Part model, mm, in its own coordinate system. Face numbers are marked on the shaded views. A direction names the side the tool comes from. Coordinates: 2 decimals unless noted, no trailing zeros. Order: outer loops, then holes, each group sorted by start corner. A loop starts at its lowest first (then second) coordinate and runs counter-clockwise, first axis right, second up.
1) Pin check, flat tips, straight feed: pin 1 Ø1.5 at (y, z) = (-3, 64) entering from +X; pin 2 Ø3 at (x, y) = (-2.5, -2.5) entering from +Z; pin 3 Ø1.5 at (y, z) = (9, 65) entering from -X. Stop position of each tip, or through.
2) Cut at B-B (z = 16). List the corners of the cut face in (x, y), and give its area (3 significant figures).
3) Mould opens along Z. For the marked faces 1, 2 and 3 say: +Z half, -Z half, draft (parallel to the pull), parting line (faces both ways), or undercut.
4) Cut at A-A (x = -23.5). List the corners of the cut face in (y, z), and give its area (3 significant figures).
5) Cut at C-C (y = 0). List the corners of the cut face in (x, z).
6) Tool access for the marked faces 4 and 5: list every direction of +Z, -Z, +X, -X, +Y, -Y with a clear straight run to the whole face (end or side of a thin tool).
7) Wall check: L1, parallel to Y at x = 18, z = -2.3; L2, parallel to X at y = 7.5, z = 4; L3, parallel to Z at x = 12, y = -9. Give the ranges that are in metal, low to high.
8) Cut at D-D (x = 18). List the corners of the cut face in (y, z).
```python
from build123d import *

# Parameters (mm, degrees)
SKETCH1_W                  = 50
SKETCH1_H                  = 50
BASE_FLANGE1_DEPTH         = 3
EDGE_FLANGE1_DEPTH         = 50
EDGE_FLANGE2_DEPTH         = 50
EDGE_FLANGE3_DEPTH         = 50
EDGE_FLANGE4_DEPTH         = 50
F_6_0_204_DIAMETER_SLOT1_D = 5.1816


# Sheet-metal steps are written as plain solids
with BuildPart() as part:
    # Sketch1 → Base-Flange1 (new body)
    with BuildSketch(Plane.XY):
        Rectangle(SKETCH1_W, SKETCH1_H)
    extrude(amount=-BASE_FLANGE1_DEPTH)

    # Edge-Flange1 section (across the edge) → Edge-Flange1 (add)
    with BuildSketch(Plane(origin=(28, -25, 0), x_dir=(-1, 0, 0), z_dir=(0, 1, 0))):
        with BuildLine():
            Line((-3, 3), (-3, 60))
            Line((-3, 60), (0, 60))
            Line((0, 60), (0, 3))
            ThreePointArc((0, 3), (0.878679656, 0.878679656), (3, 0))
            Line((3, 0), (3, -3))
            ThreePointArc((3, -3), (-1.242640687, -1.242640687), (-3, 3))
        make_face()
    extrude(amount=EDGE_FLANGE1_DEPTH)

    # Edge-Flange2 section (across the edge) → Edge-Flange2 (add)
    with BuildSketch(Plane(origin=(-28, 25, 0), x_dir=(1, 0, 0), z_dir=(0, -1, 0))):
        with BuildLine():
            Line((-3, 3), (-3, 60))
            Line((-3, 60), (0, 60))
            Line((0, 60), (0, 3))
            ThreePointArc((0, 3), (0.878679656, 0.878679656), (3, 0))
            Line((3, 0), (3, -3))
            ThreePointArc((3, -3), (-1.242640687, -1.242640687), (-3, 3))
        make_face()
    extrude(amount=EDGE_FLANGE2_DEPTH)

    # Edge-Flange3 section (across the edge) → Edge-Flange3 (add)
    with BuildSketch(Plane(origin=(-28, 25, 63), x_dir=(0, 0, -1), z_dir=(0, -1, 0))):
        with BuildLine():
            Line((-3, 3), (-3, 17))
            Line((-3, 17), (0, 17))
            Line((0, 17), (0, 3))
            ThreePointArc((0, 3), (0.878679656, 0.878679656), (3, 0))
            Line((3, 0), (3, -3))
            ThreePointArc((3, -3), (-1.242640687, -1.242640687), (-3, 3))
        make_face()
    extrude(amount=EDGE_FLANGE3_DEPTH)

    # Edge-Flange4 section (across the edge) → Edge-Flange4 (add)
    with BuildSketch(Plane(origin=(28, -25, 63), x_dir=(0, 0, -1), z_dir=(0, 1, 0))):
        with BuildLine():
            Line((-3, 3), (-3, 17))
            Line((-3, 17), (0, 17))
            Line((0, 17), (0, 3))
            ThreePointArc((0, 3), (0.878679656, 0.878679656), (3, 0))
            Line((3, 0), (3, -3))
            ThreePointArc((3, -3), (-1.242640687, -1.242640687), (-3, 3))
        make_face()
    extrude(amount=EDGE_FLANGE4_DEPTH)

    # #6 (0.204) Diameter Slot1 (through all)
    with Locations(Plane.XY.offset(66)):
        with Locations((-18, 15), (-18, -15), (18, 15), (18, -15)):
            Hole(F_6_0_204_DIAMETER_SLOT1_D / 2)


solid = part.part
```
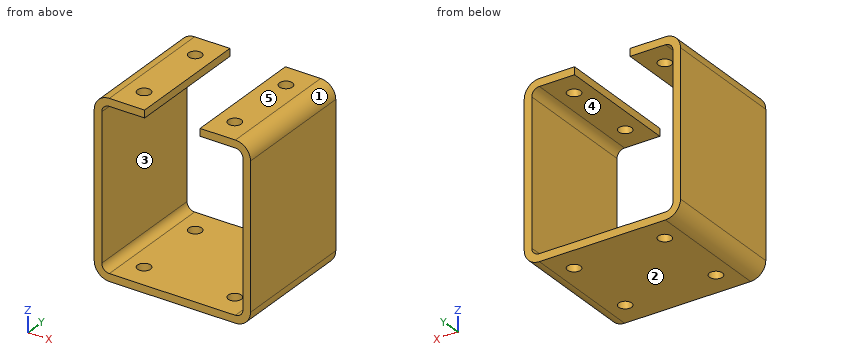
Geometry check:
1. pin 1: stops at x = 30.04
1. pin 2: stops at z = 0
1. pin 3: stops at x = -29.24
2. outline: (-31, -25) - (-28, -25) - (-28, 25) - (-31, 25) - close; (28, -25) - (31, -25) - (31, 25) - (28, 25) - close
2. area: 300 mm2
3. face 1: +Z half
3. face 2: -Z half
3. face 3: undercut
4. outline: (-25, -3) - (25, -3) - (25, 0) - (-25, 0) - close; (-25, 63) - (25, 63) - (25, 66) - (-25, 66) - close
4. area: 300 mm2
5. outline: (-31, 3) arc R6 ccw to (-25, -3) - (25, -3) arc R6 ccw to (31, 3) - (31, 60) arc R6 ccw to (25, 66) - (11, 66) - (11, 63) - (25, 63) arc R3 cw to (28, 60) - (28, 3) arc R3 cw to (25, 0) - (-25, 0) arc R3 cw to (-28, 3) - (-28, 60) arc R3 cw to (-25, 63) - (-11, 63) - (-11, 66) - (-25, 66) arc R6 ccw to (-31, 60) - close
6. face 4: +Y, -Y
6. face 5: +Z, +X, -X, +Y, -Y
7. L1: y = -25 to -17.59, -12.41 to 12.41, 17.59 to 25
7. L2: x = -31 to -28, 28 to 31
7. L3: z = -3 to 0, 63 to 66
8. outline: (-25, -3) - (-17.59, -3) - (-17.59, 0) - (-25, 0) - close; (-25, 63) - (-17.59, 63) - (-17.59, 66) - (-25, 66) - close; (-12.41, -3) - (12.41, -3) - (12.41, 0) - (-12.41, 0) - close; (-12.41, 63) - (12.41, 63) - (12.41, 66) - (-12.41, 66) - close; (17.59, -3) - (25, -3) - (25, 0) - (17.59, 0) - close; (17.59, 63) - (25, 63) - (25, 66) - (17.59, 66) - close
